```python
from build123d import *

# Parameters (mm, degrees)
ESBO_O2_R                = 0.25
RESSALTO_EXTRUS_O1_DEPTH = 10


with BuildPart() as part:
    # Esboço1 → Revolução1 (revolve)
    with BuildSketch(Plane.XY, mode=Mode.PRIVATE) as revolu_o1_sk:
        with BuildLine():
            Line((0, 4), (0.25, 4))
            ThreePointArc((0.25, 4), (0.780330086, 3.780330086), (1, 3.25))
            Line((1, 3.25), (1, 1))
            Line((1, 1), (1.5, 1))
            Line((1.5, 1), (1.5, 0))
            Line((1.5, 0), (0, 0))
            Line((0, 0), (0, 4))
        make_face()
    revolve(revolu_o1_sk.sketch.rotate(Axis((0, 0, 0), (0, 1, 0)), 90), axis=Axis((0, 0, 0), (0, 1, 0)))

    # Esboço2 → Ressalto-extrusão1 (add)
    with BuildSketch(Plane.XZ):
        with Locations(Location((-1.25, 0, 0), (0, 0, 179.998224755))):
            Circle(ESBO_O2_R)
        with Locations(Location((1.25, 0, 0), (0, 0, 90))):
            Circle(ESBO_O2_R)
    extrude(amount=RESSALTO_EXTRUS_O1_DEPTH)


solid = part.part
```
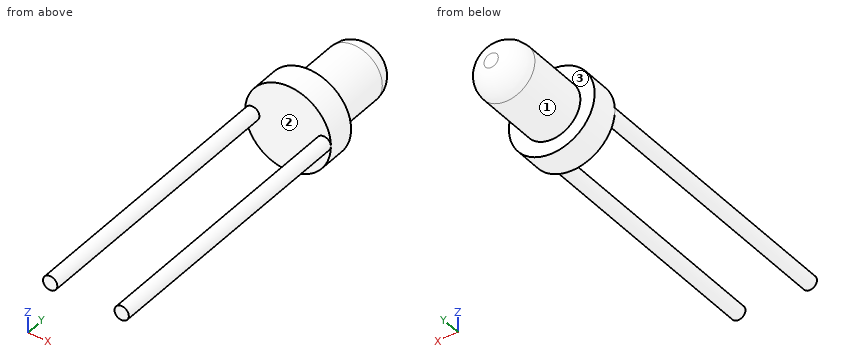
Check sheet for the modelled part. Datum: model origin and axes. Units: mm. Face numbers are marked on the shaded views. Coordinates: 2 decimals unless noted, no trailing zeros. Write each loop counter-clockwise with the first axis right and the second up, starting at its lowest first coordinate (ties: lowest second). Pieces come first, ordered by that corner, then holes. Notation, with made-up numbers: M 15.25,76.5 L 32.25,76.5 A31 cw 32.25,109.5 Z; hole C 84.25,29.25 d9. An arc over 180 degrees is marked long. Use one line per item in the form item = value.
Item 1: Sectioned sample at D-D, the plane x = 1.25. Record the cut outline in (y, z), and give its area (3 significant figures).
Answer below:
outline = M -10,-0.25 L 0,-0.25 L 0,-0.83 L 1,-0.83 L 1,0.83 L 0,0.83 L 0,0.25 L -10,0.25 Z
area = 6.66 mm^2
Item 2: Material ranges on L1, parallel to Y at x = -0.4, z = 1.3; L2, parallel to X at y = -8, z = -0.1; L3, parallel to X at y = 3, z = -0.05, recorded low to high. Write a range as from..to.
Answer below:
L1 = 0..1
L2 = -1.48..-1.02, 1.02..1.48
L3 = -1..1
Item 3: Sectioned sample at C-C, the plane y = 2.75. Record the cut outline in (x, z).
Answer below:
outline = C 0,0 d2
Item 4: Sectioned sample at B-B, the plane x = -1.15. Record the cut outline in (y, z), and give its area (3 significant figures).
Answer below:
outline = M -10,-0.23 L 0,-0.23 L 0,-0.96 L 1,-0.96 L 1,0.96 L 0,0.96 L 0,0.23 L -10,0.23 Z
area = 6.51 mm^2
Item 5: Gauge pin test, flat ends, axial feed: pin 1 Ø0.9 at (x, z) = (-0.5, 0) entering from +Y; pin 2 Ø1 at (x, z) = (-1, -1) entering from -Y. Record the tip position at first contact, or that the pin passes through.
Answer below:
pin_1 = 4
pin_2 = 0
Item 6: Sectioned sample at A-A, the plane y = -7. Record the cut outline in (x, z), and give its area (3 significant figures).
Answer below:
outline = C -1.25,0 d0.5; C 1.25,0 d0.5
area = 0.393 mm^2
Item 7: Release check for a two-part mould opening along Y. For the marked faces 1, 2 and 3 record: pulls with the +Y half, pulls with the -Y half, needs draft (parallel to the pull), parting line crosses it, or undercut.
Answer below:
face_1 = needs draft
face_2 = pulls with the -Y half
face_3 = pulls with the +Y half
